```python
from build123d import *

# Parameters (mm, degrees)
F1_DEPTH       = 10
F3_DEPTH       = 7.5
F5_R           = 4.25
F6_DEPTH       = 30
F8_D           = 4
F8_DEPTH       = 8.5
F8_CBORE_D     = 7.2
F8_CBORE_DEPTH = 5.5
F8_TIP         = 1.2017212381
F9_D           = 3.5
F9_DEPTH       = 7
F9_CBORE_D     = 7.2
F9_CBORE_DEPTH = 3.5
F9_TIP         = 1.0515060833
F10_R          = 5
F11_R          = 5
F12_W          = 3.5
F12_H          = 12.5
F13_DEPTH      = 150.001
F7_R           = 1.1
F14_DEPTH      = 18
F15_T1_DEPTH   = 109.6192794117
F16_T1_DEPTH   = 109.6192794117


# Not quite as in the source:
# - a fillet or chamfer that OpenCascade refuses, or shapes differently, is made with other operations: its cross-section is extruded or revolved along the edge and cut away or added


with BuildPart() as f1:
    # F0 (on Front) → F1 (new body)
    with BuildSketch(Plane.XZ):
        Polygon((75, 12.5), (-75, 12.5), (-75, -12.5), (-50.5, -12.5), (75, -12.5), align=None)
    extrude(amount=-F1_DEPTH)

    # F2 (on face) → F3 (cut)
    with BuildSketch(Plane.XZ):
        with BuildLine():
            Line((-50.5, 0), (-50.5, -12.5))
            Line((-50.5, -12.5), (-29.5, -12.5))
            Line((-29.5, -12.5), (-29.5, 0))
            ThreePointArc((-29.5, 0), (-29.5018489924, 1.0611519764), (-29.616133488, 2.116133488))
            ThreePointArc((-29.616133488, 2.116133488), (-32.4157560185, 7.5842439815), (-37.883866512, 10.383866512))
            ThreePointArc((-37.883866512, 10.383866512), (-38.9388480236, 10.4981510076), (-40, 10.5))
            ThreePointArc((-40, 10.5), (-46.7951402173, 8.2937242033), (-50.383866512, 2.116133488))
            ThreePointArc((-50.383866512, 2.116133488), (-50.4981510076, 1.0611519764), (-50.5, 0))
        make_face()
        with BuildLine():
            ThreePointArc((29.616133488, 2.116133488), (29.5018489924, 1.0611519764), (29.5, 0))
            Line((29.5, 0), (29.5, -12.5))
            Line((29.5, -12.5), (50.5, -12.5))
            Line((50.5, -12.5), (50.5, 0))
            ThreePointArc((50.5, 0), (50.4981510076, 1.0611519764), (50.383866512, 2.116133488))
            ThreePointArc((50.383866512, 2.116133488), (47.5842439815, 7.5842439815), (42.116133488, 10.383866512))
            ThreePointArc((42.116133488, 10.383866512), (41.0611519764, 10.4981510076), (40, 10.5))
            ThreePointArc((40, 10.5), (38.9388480236, 10.4981510076), (37.883866512, 10.383866512))
            ThreePointArc((37.883866512, 10.383866512), (32.4157560185, 7.5842439815), (29.616133488, 2.116133488))
        make_face()
        with BuildLine():
            Line((-65, -12.5), (-59.4149563834, -12.5))
            Line((-59.4149563834, -12.5), (-50.5, -12.5))
            Line((-50.5, -12.5), (-50.5, 0))
            ThreePointArc((-50.5, 0), (-50.4981510076, 1.0611519764), (-50.383866512, 2.116133488))
            Line((-50.383866512, 2.116133488), (-65, -12.5))
        make_face()
        Polygon((-29.5, 0), (-29.5, -12.5), (-15, -12.5), (-27.5, 0), align=None)
        with BuildLine():
            ThreePointArc((-29.616133488, 2.116133488), (-29.5018489924, 1.0611519764), (-29.5, 0))
            Line((-29.5, 0), (-27.5, 0))
            Line((-27.5, 0), (-29.616133488, 2.116133488))
        make_face()
        Polygon((27.5, 0), (15, -12.5), (17, -12.5), (19.8756534234, -12.5), (29.5, -12.5), (29.5, 0), align=None)
        with BuildLine():
            Line((29.616133488, 2.116133488), (27.5, 0))
            Line((27.5, 0), (29.5, 0))
            ThreePointArc((29.5, 0), (29.5018489924, 1.0611519764), (29.616133488, 2.116133488))
        make_face()
        with BuildLine():
            Line((50.5, 0), (52.5, 0))
            Line((52.5, 0), (50.383866512, 2.116133488))
            ThreePointArc((50.383866512, 2.116133488), (50.4981510076, 1.0611519764), (50.5, 0))
        make_face()
        Polygon((62.5, -10.8300764114), (62.5, -10), (52.5, 0), (50.5, 0), (50.5, -12.5), (62.5, -12.5), align=None)
        Polygon((62.5, -12.5), (65, -12.5), (62.5, -10), (62.5, -10.8300764114), align=None)
    extrude(amount=-F3_DEPTH, mode=Mode.SUBTRACT)

    # F4: F1 across face


with BuildPart() as f1_1:
    add(f1.part)
    add(f1.part.mirror(Plane.XZ))

    # F5 (on face) → F6 (cut)
    with BuildSketch(Plane.XY.offset(12.5)):
        Circle(F5_R)
    extrude(amount=-F6_DEPTH, mode=Mode.SUBTRACT)

    # F8
    with Locations(Plane.XZ.offset(10)):
        with Locations((-70.5, -8.5), (-9.5, -8.5), (9.5, -8.5), (70.5, -8.5)):
            CounterBoreHole(F8_D / 2, F8_CBORE_D / 2, F8_CBORE_DEPTH, depth=F8_DEPTH)
            with Locations((0, 0, -(F8_DEPTH + F8_TIP / 2))):  # 118° drill point
                Cone(0, F8_D / 2, F8_TIP, mode=Mode.SUBTRACT)

    # F9
    with Locations(Plane.XZ.offset(10)):
        with Locations((0, 7.5)):
            CounterBoreHole(F9_D / 2, F9_CBORE_D / 2, F9_CBORE_DEPTH, depth=F9_DEPTH)
            with Locations((0, 0, -(F9_DEPTH + F9_TIP / 2))):  # 118° drill point
                Cone(0, F9_D / 2, F9_TIP, mode=Mode.SUBTRACT)

    # F10
    f10_edges = [f1_1.edges().sort_by_distance(p)[0] for p in [
        (-29.616133, 0, 2.116133),
    ]]
    fillet(f10_edges, radius=F10_R)

    # F11
    f11_edges = [f1_1.edges().sort_by_distance(p)[0] for p in [
        (-50.383867, 0, 2.116133),
    ]]
    fillet(f11_edges, radius=F11_R)

    # F12 (on face) → F13 (cut, through all)
    with BuildSketch(Plane.YZ.offset(75)):
        with Locations((0, -6.25)):
            Rectangle(F12_W, F12_H)
        Polygon((-7.5, 0), (-1.75, 0), (1.75, 0), (7.5, 0), (7.5, 3), (-7.5, 3), align=None)
    extrude(amount=-F13_DEPTH, mode=Mode.SUBTRACT)

    # F7 (on face) → F14 (cut)
    with BuildSketch(Plane.XZ.offset(10)):
        with Locations((-70.5, -8.5)):
            Circle(F7_R)
        with Locations((-9.5, -8.5)):
            Circle(F7_R)
        with Locations((9.5, -8.5)):
            Circle(F7_R)
        with Locations((70.5, -8.5)):
            Circle(F7_R)
    extrude(amount=-F14_DEPTH, mode=Mode.SUBTRACT)

    # F15: chamfer of 10 x 17.3205080757 on 1 edges, made by hand

    # F15_s2 → F15_t1 (cut)
    with BuildSketch(Plane.XZ.offset(-54.8096397058)):
        Polygon((-75, -4.8205080757), (-65, 12.5), (-75, 12.5), align=None)
    extrude(amount=F15_T1_DEPTH, mode=Mode.SUBTRACT)

    # F16: chamfer of 10 x 17.3205080757 on 1 edges, made by hand

    # F16_s2 → F16_t1 (cut)
    with BuildSketch(Plane.XZ.offset(-54.8096397058)):
        Polygon((75, -4.8205080757), (65, 12.5), (75, 12.5), align=None)
    extrude(amount=F16_T1_DEPTH, mode=Mode.SUBTRACT)


solid = f1_1.part
```
CAD build for the part. Positions are in the model's coordinates, mm. A direction names the side the tool comes from. Coordinates: 2 decimals unless noted, no trailing zeros. Write each loop counter-clockwise with the first axis right and the second up, starting at its lowest first coordinate (ties: lowest second). Pieces come first, ordered by that corner, then holes. Notation, with made-up numbers: (-33.75, -22.5) -> (-12.75, -22.5) arc R28 cw to (-12.75, 4.5) -> close; hole circle Ø4 at (78, -14). An arc over 180 degrees is marked (long way). Use CSV: the item, a comma, the result in double quotes. Start each with the question number.
Item 1: Band-saw the part on A-A, the plane x = 59. Write the cut outline in (y, z).
Item 2: Drop flat-ended pins along their axis: P1, Ø4, axis at y = -2.5, z = 0.5, coming from the -X side; P2, Ø7.5, axis at x = 0, y = 0, coming from the -Z side; P3, Ø10, axis at x = -39, y = 0.5, coming from the -Z side; P4, Ø1, axis at x = -55, y = -3.5, coming from the -Z side. Give the stop position or say it passes through.
Item 3: Band-saw the part on C-C, the plane x = -26. Write the cut outline in (y, z).
Item 4: Tool access for faces 5 (the flat face through (21.3, -4.6, -6.2)), 6 (the flat face through (60, 0, 3)), 7 (the flat face through (-1, 7.5, 2)), 8 (the flat face through (-7.95, -4.5, -10.05)), 9 (the flat face through (13, -1.75, -5)): list every direction of +Z, -Z, +X, -X, +Y, -Y with a clear straight run to the whole face (end or side of a thin tool).
Item 5: Band-saw the part on D-D, the plane x = 44. Write the cut outline in (y, z), plus the area to 3 significant figures.
Item 6: Band-saw the part on B-B, the plane z = 7.5. Write the cut outline in (x, y).
Item 7: Two-plate mould, pull along X, no slides. Class faces 1 (the flat face through (62, -5, 0)), 2 (the flat face through (11.05, -4.5, -10.05)), 3 (the flat face through (-58.7, -4.6, -6.2)), 4 (the flat face through (-75, -6, -9)): +X half, -X half, draft (parallel to the pull), parting line (faces both ways), or undercut.
Item 8: Wall check: probe 1 along Z at (x, y) = (-9.5, 4); probe 2 along Z at (x, y) = (9.5, -2.3); probe 3 along Y at (x, z) = (-4, -1.25). Give the ranges that are in metal, low to high.
Response values:
1,outline,"(-10, -12.5) -> (-7.5, -12.5) -> (-7.5, -6.5) -> (-1.75, -6.5) -> (-1.75, 0) -> (-7.5, 0) -> (-7.5, 3) -> (7.5, 3) -> (7.5, 0) -> (1.75, 0) -> (1.75, -6.5) -> (7.5, -6.5) -> (7.5, -12.5) -> (10, -12.5) -> (10, 12.5) -> (-10, 12.5) -> close"
2,P1,"stops at x = -73.08"
2,P2,"passes through"
2,P3,"stops at z = 8.87"
2,P4,"stops at z = -3"
3,outline,"(-10, -12.5) -> (-7.5, -12.5) -> (-7.5, -1.5) -> (-1.75, -1.5) -> (-1.75, 0) -> (-7.5, 0) -> (-7.5, 3) -> (7.5, 3) -> (7.5, 0) -> (1.75, 0) -> (1.75, -1.5) -> (7.5, -1.5) -> (7.5, -12.5) -> (10, -12.5) -> (10, 12.5) -> (-10, 12.5) -> close"
4,face 5,"-Z"
4,face 6,"+X, -X"
4,face 7,"none"
4,face 8,"-Y"
4,face 9,"-Z, +X, -X"
5,outline,"(-10, -12.5) -> (-7.5, -12.5) -> (-7.5, 9.89) -> (7.5, 9.89) -> (7.5, -12.5) -> (10, -12.5) -> (10, 12.5) -> (-10, 12.5) -> close"
5,area,"164 mm2"
6,outline,"(-67.89, -10) -> (-3.6, -10) -> (-3.6, -6.5) -> (-1.75, -6.5) -> (-1.75, -3.87) arc R4.25 cw (long way) to (1.75, -3.87) -> (1.75, -6.5) -> (3.6, -6.5) -> (3.6, -10) -> (67.89, -10) -> (67.89, 10) -> (-67.89, 10) -> close; hole (-47.67, -7.5) -> (-32.33, -7.5) -> (-32.33, 7.5) -> (-47.67, 7.5) -> close; hole (32.33, -7.5) -> (47.67, -7.5) -> (47.67, 7.5) -> (32.33, 7.5) -> close"
7,face 1,"draft"
7,face 2,"undercut"
7,face 3,"undercut"
7,face 4,"-X half"
8,probe 1,"z = -12.5 to -9.6, -7.4 to 0, 3 to 12.5"
8,probe 2,"z = -12.5 to -10.5, -6.5 to 0, 3 to 12.5"
8,probe 3,"y = -10 to -1.75, 1.75 to 10"
